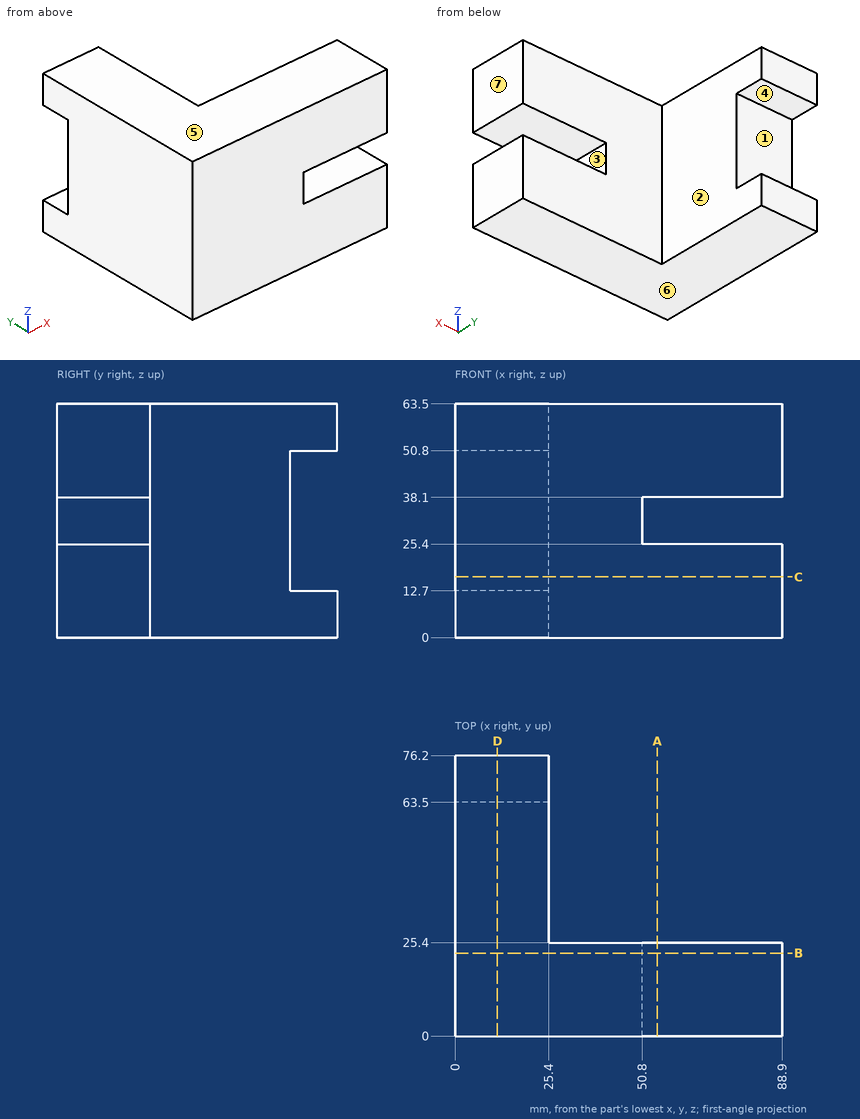
The figure shows three views and two pictorial views of one solid part (mm, origin at its lowest corner). Answer the questions. A direction names the side the tool comes from. Coordinates: 2 decimals unless noted, no trailing zeros. Loops run counter-clockwise (first coordinate to the right, second up) from the corner with the lowest first, then second, coordinate; pieces in that order, holes last. Notation, with made-up numbers: (63.5, 42.25) -> (83.5, 42.25) arc R15 cw to (83.5, 48.25) -> close; hole circle Ø3 at (72.25, -15). An arc over 180 degrees is marked (long way). Use one line per item in the form item = value. Start each with the question number.
Item 1: The part is cut by section D-D on x = 11.5. Determine the outline of the cut face in (y, z), then the cut area to 3 significant figures.
Item 2: A tool of negligible diameter and unlimited length cuts with its end or side. For the marked faces 1, 2 and 3, from which of +Z, -Z, +X, -X, +Y, -Y can it reach the whole face along a straight path? Write none if from no direction.
Item 3: Consider L1, parallel to Y at x = 37.5, z = 11; L2, parallel to Z at x = 11.5, y = 67. Determine where each line is inside the solid, lowest interval first. Write a range as [from, to].
Item 4: The mould has two halves that part along Z. Classify the marked faces 4, 5, 6 and 7: released by +Z, released by -Z, zero draft, split by the parting line, or undercut.
Item 5: Flat-ended cylindrical pins translate along their axes: pin 1 Ø19 at (x, z) = (56, 30.5) entering from +Y; pin 2 Ø10 at (y, z) = (16.5, 33) entering from +X. Find the tip coordinate at first contact, or state that the pin passes through.
Item 6: The part is cut by section C-C on z = 16.5. Determine the outline of the cut face in (x, y).
Item 7: The part is cut by section B-B on y = 22.5. Determine the outline of the cut face in (x, z), then the cut area to 3 significant figures.
Item 8: The part is cut by section A-A on x = 55. Determine the outline of the cut face in (y, z).
Answer key:
q1.outline = (0, 0) -> (76.2, 0) -> (76.2, 12.7) -> (63.5, 12.7) -> (63.5, 50.8) -> (76.2, 50.8) -> (76.2, 63.5) -> (0, 63.5) -> close
q1.area = 4,350 mm2
q2.face_1 = +X, -X, +Y
q2.face_2 = +Z, -Z, +X, +Y
q2.face_3 = +X, +Y, -Y
q3.L1 = [0, 25.4]
q3.L2 = [0, 12.7], [50.8, 63.5]
q4.face_4 = undercut
q4.face_5 = released by +Z
q4.face_6 = released by -Z
q4.face_7 = zero draft
q5.pin_1 = 25.4
q5.pin_2 = 50.8
q6.outline = (0, 0) -> (88.9, 0) -> (88.9, 25.4) -> (25.4, 25.4) -> (25.4, 63.5) -> (0, 63.5) -> close
q7.outline = (0, 0) -> (88.9, 0) -> (88.9, 25.4) -> (50.8, 25.4) -> (50.8, 38.1) -> (88.9, 38.1) -> (88.9, 63.5) -> (0, 63.5) -> close
q7.area = 5,160 mm2
q8.outline = (0, 0) -> (25.4, 0) -> (25.4, 25.4) -> (0, 25.4) -> close; (0, 38.1) -> (25.4, 38.1) -> (25.4, 63.5) -> (0, 63.5) -> close
